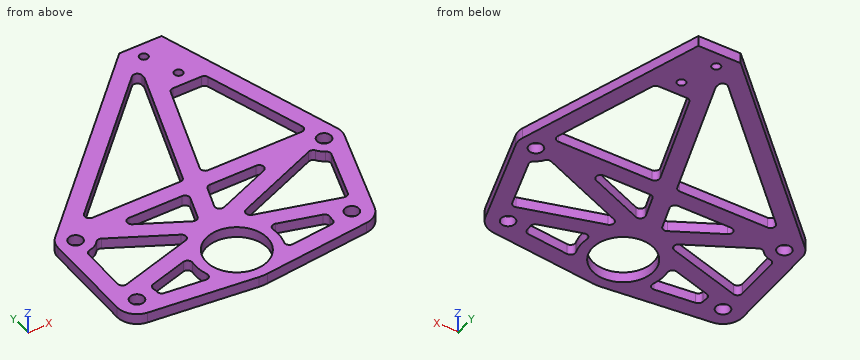
```python
from build123d import *

# Parameters (mm, degrees)
SKETCH1_R           = 3.302
SKETCH1_R_2         = 14.2748
SKETCH1_R_3         = 2
BOSS_EXTRUDE1_DEPTH = 5
FILLET1_R           = 2.2


with BuildPart() as part:
    # Sketch1 → Boss-Extrude1 (new body)
    with BuildSketch(Plane.XY):
        with BuildLine():
            Line((49.732074359, 129.130431425), (29.732074359, 129.130431425))
            Line((29.732074359, 129.130431425), (-54.986003567, 45.902692248))
            ThreePointArc((-54.986003567, 45.902692248), (-56.787195673, 43.277388838), (-57.467824457, 40.167203079))
            Line((-57.467824457, 40.167203079), (-58.467571363, -4.260299734))
            ThreePointArc((-58.467571363, -4.260299734), (-56.161422432, -10.602936869), (-50.173941362, -13.717008024))
            Line((-50.173941362, -13.717008024), (-1.066715703, -19.05931292))
            ThreePointArc((-1.066715703, -19.05931292), (0.992574977, -19.172351986), (3.052155178, -19.06471679))
            Line((3.052155178, -19.06471679), (53.413821776, -13.719615927))
            ThreePointArc((53.413821776, -13.719615927), (58.261915472, -11.718027487), (61.25647558, -7.411871598))
            Line((61.25647558, -7.411871598), (76.182819246, 37.354437047))
            ThreePointArc((76.182819246, 37.354437047), (76.608419263, 39.876139592), (76.246305111, 42.407738382))
            Line((76.246305111, 42.407738382), (49.732074359, 129.130431425))
        make_face()
        with Locations((-49.167925641, -4.469568575)):
            Circle(SKETCH1_R, mode=Mode.SUBTRACT)
        with BuildLine():
            Line((-15.743011398, -9.415499117), (-40.152332132, -6.760044))
            ThreePointArc((-40.152332132, -6.760044), (-39.904287902, -3.625637398), (-40.714646148, -0.587652835))
            Line((-40.714646148, -0.587652835), (-17.187009107, 6.434930438))
            ThreePointArc((-17.187009107, 6.434930438), (-18.177445963, -1.64628978), (-15.743011398, -9.415499117))
        make_face(mode=Mode.SUBTRACT)
        with Locations((1.017863078, 0.102431425)):
            Circle(SKETCH1_R_2, mode=Mode.SUBTRACT)
        with BuildLine():
            ThreePointArc((-49.656497245, 31.692820081), (-45.010872906, 32.79418647), (-41.740102305, 36.27224528))
            Line((-41.740102305, 36.27224528), (-7.597542604, 17.645980927))
            Line((-7.597542604, 17.645980927), (-50.259137287, 4.912249924))
            Line((-50.259137287, 4.912249924), (-49.656497245, 31.692820081))
        make_face(mode=Mode.SUBTRACT)
        with Locations((-49.167925641, 39.980431425)):
            Circle(SKETCH1_R, mode=Mode.SUBTRACT)
        Polygon((-32.386395914, 40.282431425), (4.475234555, 40.282431425), (-1.533823666, 23.450999579), align=None, mode=Mode.SUBTRACT)
        with BuildLine():
            ThreePointArc((60.530999596, 37.07253437), (62.657762713, 33.896971725), (65.981819268, 32.010714193))
            Line((65.981819268, 32.010714193), (56.592331805, 3.850254859))
            ThreePointArc((56.592331805, 3.850254859), (55.825298544, 4.191449473), (55.030627874, 4.462101125))
            Line((55.030627874, 4.462101125), (12.139397937, 16.940748464))
            Line((12.139397937, 16.940748464), (60.530999596, 37.07253437))
        make_face(mode=Mode.SUBTRACT)
        with BuildLine():
            ThreePointArc((17.753705258, -9.459446089), (20.216903145, -1.60483995), (19.178334944, 6.561160143))
            Line((19.178334944, 6.561160143), (43.95204944, -0.646430941))
            ThreePointArc((43.95204944, -0.646430941), (43.16663603, -3.645641046), (43.410501788, -6.736379627))
            Line((43.410501788, -6.736379627), (17.753705258, -9.459446089))
        make_face(mode=Mode.SUBTRACT)
        with Locations((52.432074359, -4.469568575)):
            Circle(SKETCH1_R, mode=Mode.SUBTRACT)
        Polygon((12.969784548, 40.282431425), (47.419131213, 40.282431425), (6.960726327, 23.450999579), align=None, mode=Mode.SUBTRACT)
        with Locations((68.307074359, 39.980431425)):
            Circle(SKETCH1_R, mode=Mode.SUBTRACT)
        Polygon((-41.148197142, 48.282431425), (29.732074359, 117.915795328), (29.732074359, 111.027090937), (7.331347226, 48.282431425), align=None, mode=Mode.SUBTRACT)
        Polygon((66.084655222, 48.282431425), (15.825897219, 48.282431425), (33.979349356, 99.130431425), (50.538601957, 99.130431425), align=None, mode=Mode.SUBTRACT)
        with Locations((36.732074359, 122.130431425)):
            Circle(SKETCH1_R_3, mode=Mode.SUBTRACT)
        with Locations((42.732074359, 106.130431425)):
            Circle(SKETCH1_R_3, mode=Mode.SUBTRACT)
    extrude(amount=BOSS_EXTRUDE1_DEPTH)

    # Fillet1
    fillet1_edges = [part.edges().sort_by_distance(p)[0] for p in [
        (43.95204944, -0.646430941, 2.5),
        (43.410501788, -6.736379627, 2.5),
        (-40.152332132, -6.760044, 2.5),
        (-40.714646148, -0.587652835, 2.5),
        (-41.148197142, 48.282431425, 2.5),
        (7.331347226, 48.282431425, 2.5),
        (66.084655222, 48.282431425, 2.5),
        (6.960726327, 23.450999579, 2.5),
        (47.419131213, 40.282431425, 2.5),
        (-49.656497245, 31.692820081, 2.5),
        (-41.740102305, 36.27224528, 2.5),
        (-50.259137287, 4.912249924, 2.5),
        (-32.386395914, 40.282431425, 2.5),
        (4.475234555, 40.282431425, 2.5),
        (12.969784548, 40.282431425, 2.5),
        (12.139397937, 16.940748464, 2.5),
        (60.530999596, 37.07253437, 2.5),
        (65.981819268, 32.010714193, 2.5),
        (56.592331805, 3.850254859, 2.5),
        (17.753705258, -9.459446089, 2.5),
        (19.178334944, 6.561160143, 2.5),
        (-15.743011398, -9.415499117, 2.5),
        (-17.187009107, 6.434930438, 2.5),
        (-7.597542604, 17.645980927, 2.5),
        (-1.533823666, 23.450999579, 2.5),
        (33.979349356, 99.130431425, 2.5),
        (15.825897219, 48.282431425, 2.5),
        (50.538601957, 99.130431425, 2.5),
        (29.732074359, 117.915795328, 2.5),
        (29.732074359, 111.027090937, 2.5),
    ]]
    fillet(fillet1_edges, radius=FILLET1_R)


solid = part.part
```
Input: part model. Units: mm. Frame: model coordinates. Coordinates: 2 decimals unless noted, no trailing zeros. Write each loop counter-clockwise with the first axis right and the second up, starting at its lowest first coordinate (ties: lowest second). Pieces come first, ordered by that corner, then holes. Notation, with made-up numbers: (82, 21.25) - (120, 21.25) arc R18 ccw to (120, 45.25) - close; hole circle Ø9 at (72.25, 51.25). An arc over 180 degrees is marked (long way). Put each result on its own line as item: value. Start each with the question number.
1) Cut plane A-A (y = 10.5). Return the cut outline in (x, z), plus the area to 3 significant figures.
2) Ray query, L1, parallel to Y at x = -20.5, z = 3; L2, parallel to Y at x = -15, z = 3.9; L3, parallel to Y at x = 44, z = 4.75. Return the intervals inside material, ascending.
3) Contact query for flat-ended pins moving along their axis: pin 1 (2 mm diameter, centred on x = -23, z = 3.5, fed in from -Y); pin 2 (1.5 mm diameter, centred on x = 21, z = 2.5, fed in from -Y); pin 3 (10.5 mm diameter, centred on x = 68.31, y = 39.98, fed in from +Z); pin 4 (1.5 mm diameter, centred on x = 43.5, z = 1.5, fed in from -Y). Output: stop coordinate, or through.
4) Cut plane B-B (y = 61). Return the cut outline in (x, z).
5) Cut plane C-C (z = 1.05). State how many separate pieces and enclosed holes the cut face has, plus the area to 3 significant figures.
Resolved:
1. outline: (-58.14, 0) - (-50.13, 0) - (-50.13, 5) - (-58.14, 5) - close; (-31.54, 0) - (-8.76, 0) - (-8.76, 5) - (-31.54, 5) - close; (10.8, 0) - (34.28, 0) - (34.28, 5) - (10.8, 5) - close; (58.81, 0) - (67.23, 0) - (67.23, 5) - (58.81, 5) - close
1. area: 313 mm2
2. L1: y = -16.95 to -8.9, 5.41 to 13.79, 24.68 to 33.8, 40.28 to 48.28, 68.57 to 79.78
2. L2: y = -17.54 to 15.44, 21.68 to 30.8, 40.28 to 48.28, 73.97 to 85.19
2. L3: y = -14.72 to 7.67, 30.2 to 48.28, 99.13 to 104.58, 107.68 to 129.13
3. pin 1: stops at y = -16.78
3. pin 2: stops at y = -17.24
3. pin 3: stops at z = 5
3. pin 4: stops at y = -14.85
4. outline: (-39.62, 0) - (-28.2, 0) - (-28.2, 5) - (-39.62, 5) - close; (11.87, 0) - (20.37, 0) - (20.37, 5) - (11.87, 5) - close; (62.2, 0) - (70.56, 0) - (70.56, 5) - (62.2, 5) - close
5. separate pieces: 1
5. enclosed holes: 15
5. area: 7,230 mm2
